Autodesk Inventor part; units mm, degrees
ref_plane "Start plane" through (0, 0, 0) normal (0, 0, 1) x (1, 0, 0)
ref_plane "End plane" through (0, 0, 1000) normal (0, 0, 1) x (1, 0, 0)
ref_plane "YZ Plane" through (0, 0, 0) normal (1, 0, 0) x (0, 1, 0)
ref_plane "Start plane" through (0, 0, 0) normal (0, 0, 1) x (1, 0, 0)
ref_plane "End plane" through (0, 0, 1000) normal (0, 0, 1) x (1, 0, 0)
sketch "Sketch" plane through (0, 0, 0) normal (0, 0, 1) x (1, 0, 0)
  line L0 (-40, -34) -> (-40, 34)
  line L1 (-34, 40) -> (34, 40)
  line L2 (40, 34) -> (40, -34)
  line L3 (34, -40) -> (-34, -40)
  arc A0 (-40, -34) -> (-34, -40) centre (-34, -34) ccw
  arc A1 (40, 34) -> (34, 40) centre (34, 34) ccw
  arc A2 (-34, 40) -> (-40, 34) centre (-34, 34) ccw
  arc A3 (34, -40) -> (40, -34) centre (34, -34) ccw
  arc A4 (-34, 37) -> (-37, 34) centre (-34, 34) ccw
  line L4 (-34, 37) -> (34, 37)
  arc A5 (37, 34) -> (34, 37) centre (34, 34) ccw
  line L5 (37, 34) -> (37, -34)
  arc A6 (34, -37) -> (37, -34) centre (34, -34) ccw
  line L6 (34, -37) -> (-34, -37)
  arc A7 (-37, -34) -> (-34, -37) centre (-34, -34) ccw
  line L7 (-37, -34) -> (-37, 34)
  line L8 (0, 57.7397) -> (0, -57.7397) construction
  line L9 (-1453.6197, 0) -> (290.3864, 0) construction
  dimension "d7" = 6
  dimension "d9" = 80
  dimension "d11" = 80
  dimension "d12" = 3
  dimension "d15" = 40
  dimension "d16" = 40
extrude "Body" add sketch "Sketch" along normal up to surface (1000 mm away) from surface at 0
sketch "Sketch3" plane through (0, 0, 0) normal (0, 0, 1) x (1, 0, 0)
  line L0 (0, 0) -> (10, 0)
ref_plane "Work Plane3" through (0, 0, 0) normal (0, -1, 0) x (1, 0, 0)
sketch "Sketch5" plane through (0, 0, 0) normal (0, 1, 0) x (-1, 0, 0)
  line L0 (-40, 0) -> (-40, 1000)
  line L1 (40, 0) -> (40, 1000)
  line L2 (40, 0) -> (40, 1000)
  line L3 (40, 278.04) -> (415, 278.04) construction
  line L4 (-5.663, 299.3796) -> (835.663, 299.3796) construction
  arc A0 (-5.663, 299.3796) -> (415, 200) centre (415, 1140) ccw construction
  line L5 (-55, 379.2385) -> (885, 379.2385) construction
  arc A1 (-55, 379.2385) -> (-5.663, 299.3796) centre (34.3, 379.2385) ccw construction
  arc A2 (835.663, 299.3796) -> (885, 379.2385) centre (795.7, 379.2385) ccw
  line L6 (-55, 379.2385) -> (-55, 419.2385)
  line L7 (885, 379.2385) -> (885, 419.2385)
  line L8 (-55, 419.2385) -> (415, 419.2385) construction
  line L9 (415, 419.2385) -> (415, 0)
  arc A3 (415, 200) -> (835.663, 299.3796) centre (415, 1140) ccw
  line L10 (415, 419.2385) -> (885, 419.2385)
  point P0 (0, 0)
  dimension "d22" = 375
  dimension "d24" = 940
  dimension "d25" = 89.3
  dimension "d26" = 40
  dimension "d27" = 940
  dimension "d28" = 200
  dimension "d30" = 278.04
sketch "Sketch6" plane through (0, 0, 0) normal (0, 1, 0) x (-1, 0, 0)
  line L0 (40, 0) -> (40, 1000)
  line L1 (40, 0) -> (40, 1000)
  line L2 (-40, 0) -> (-40, 1000)
  line L3 (-40, 0) -> (-40, 1000)
  line L4 (34, 1000) -> (40, 1000)
  line L5 (40, 1000) -> (-40, 1000)
  arc A0 (-5.663, 299.3796) -> (415, 200) centre (415, 1140) ccw construction
  line L6 (40, 270.8824) -> (-40, 300)
  point P0 (0, 0)
  dimension "d34" = 110
  dimension "d36" = 300
extrude "Extrusion2" cut sketch "Sketch6" along normal through all both and the other way through all
sketch "Sketch4" plane through (0, 0, 0) normal (0, -1, 0) x (1, 0, 0)
  line L0 (-1453.3712, 0) -> (288.8952, 0)
  line L1 (-1453.3712, 1000) -> (288.8952, 1000)
  dimension "d18" = 1000
equation "\"d7\" = G_IR"
equation "\"d9\" = G_W"
equation "\"d11\" = G_H"
equation "\"d12\" = G_T"
equation "\"d15\" = 0.5 * d9"
equation "\"d16\" = 0.5 * d11"
equation "\"d3\" = G_L"
equation "\"d22\" = 0.5 * Diam_of_legs_center"
equation "\"d24\" = d27"
equation "\"d25\" = 0.095 * d27"
equation "\"d27\" = MAIN_filter_diam"
equation "\"G_W\" = 80"
equation "\"G_H\" = 80"
equation "\"G_T\" = 3"
equation "\"G_IR\" = 6"
equation "\"G_L\" = d18"
equation "\"G_OFFSET_START\" = 0"
equation "\"G_OFFSET_END\" = 0"
equation "\"MAIN_filter_diam\" = 940"
properties part number "SLM 1692 Leg tube" material "Steel, Mild"
For this review, take the finished solid that the model builds, in its own axes (mm). A direction names the side the tool comes from. Round coordinates to 2 decimals unless told otherwise and drop trailing zeros. Write each loop counter-clockwise with the first axis right and the second up, starting at its lowest first coordinate (ties: lowest second). Pieces come first, ordered by that corner, then holes. Notation, with made-up numbers: M -16.5,17.5 L 32.5,17.5 A20 cw 32.5,56.5 Z; hole C 82.25,82 d6. An arc over 180 degrees is marked long. Write item = value, one per line. Start each with the question number.
(1) We need section B-B (z = 255.5). Give the boundary of the cut face in (x, y), then the cut area to 3 significant figures.
(2) We need section C-C (x = -9). Give the boundary of the cut face in (y, z), then the cut area to 3 significant figures.
(3) For faces 1 (the face through (37, 0, 147)), 2 (the face through (-40, 0, 134)), list the 3-axis set-ups (+Z, -Z, +X, -X, +Y, -Y) from which the entire face can be reached by the end or side of a thin tool; tool diameter is ignored.
(4) The part is to be moulded in two halves that separate along X. For faces 3 (the face through (-38.289, 38.196, 134.622)), 4 (the face through (0, -37, 147)), 5 (the face through (40, 0, 148)), say which applies: +X half, -X half, draft (parallel to the pull), parting line (faces both ways), or undercut.
(5) We need section A-A (y = 24.5). Give the boundary of the cut face in (x, z), then the cut area to 3 significant figures.
(6) For line 1 along X through (y, z) = (-18.5, 85); line 2 along X through (y, z) = (0, 279), list the stretches that pass through material, from the lowest coordinate up.
Results found:
q1.outline = M -40,-34 A6 ccw -34,-40 L 34,-40 A6 ccw 40,-34 L 40,34 A6 ccw 34,40 L -34,40 A6 ccw -40,34 Z; hole M -37,-34 A3 ccw -34,-37 L 34,-37 A3 ccw 37,-34 L 37,34 A3 ccw 34,37 L -34,37 A3 ccw -37,34 Z
q1.area = 901 mm²
q2.outline = M -40,0 L -37,0 L -37,282.17 L -40,282.17 Z; M 37,0 L 40,0 L 40,282.17 L 37,282.17 Z
q2.area = 1,690 mm²
q3.face_1 = +Z, -Z
q3.face_2 = +Z, -Z, -X, +Y, -Y
q4.face_3 = -X half
q4.face_4 = undercut
q4.face_5 = +X half
q5.outline = M -40,0 L -37,0 L -37,271.97 L -40,270.88 Z; M 37,0 L 40,0 L 40,300 L 37,298.91 Z
q5.area = 1,710 mm²
q6.line_1 = -40 to -37, 37 to 40
q6.line_2 = 37 to 40
